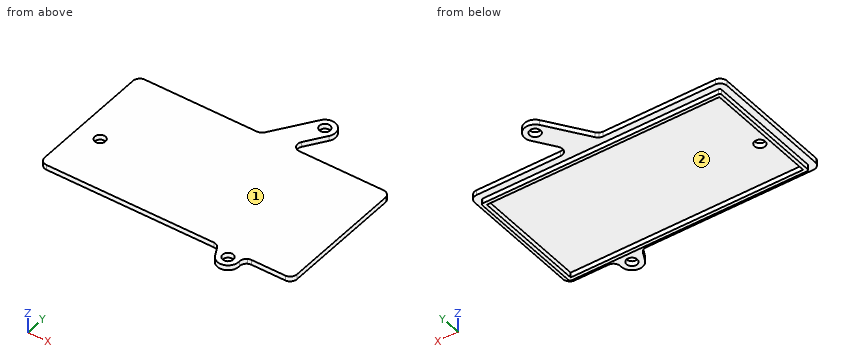
```python
from build123d import *

# Parameters (mm, degrees)
SKETCH1_W           = 69.1
SKETCH1_H           = 34.1
BOSS_EXTRUDE1_DEPTH = 1.5
BOSS_EXTRUDE2_DEPTH = 1.5
SKETCH3_R           = 1.6
BOSS_EXTRUDE3_DEPTH = 1.5
SKETCH3_2_R         = 1.6
CUT_EXTRUDE1_DEPTH  = 85.057646739


with BuildPart() as part:
    # Sketch1 → Boss-Extrude1 (new body)
    with BuildSketch(Plane.XY.offset(19)):
        with BuildLine():
            Line((4.325559412, 33.249665151), (-65.674440588, 33.249665151))
            ThreePointArc((-65.674440588, 33.249665151), (-66.063349318, 33.088573881), (-66.224440588, 32.699665151))
            Line((-66.224440588, 32.699665151), (-66.224440588, -2.300334849))
            ThreePointArc((-66.224440588, -2.300334849), (-66.063349318, -2.689243578), (-65.674440588, -2.850334849))
            Line((-65.674440588, -2.850334849), (4.325559412, -2.850334849))
            ThreePointArc((4.325559412, -2.850334849), (4.714468141, -2.689243578), (4.875559412, -2.300334849))
            Line((4.875559412, -2.300334849), (4.875559412, 32.699665151))
            ThreePointArc((4.875559412, 32.699665151), (4.714468141, 33.088573881), (4.325559412, 33.249665151))
        make_face()
        with Locations((-30.674440588, 15.199665151)):
            Rectangle(SKETCH1_W, SKETCH1_H, mode=Mode.SUBTRACT)
    extrude(amount=-BOSS_EXTRUDE1_DEPTH)

    # Sketch2 → Boss-Extrude2 (add)
    with BuildSketch(Plane.XY.offset(19)):
        with BuildLine():
            Line((6.825559412, -2.800334849), (6.825559412, 33.199665151))
            ThreePointArc((6.825559412, 33.199665151), (6.239772974, 34.613878714), (4.825559412, 35.199665151))
            Line((4.825559412, 35.199665151), (-66.174440588, 35.199665151))
            ThreePointArc((-66.174440588, 35.199665151), (-67.588654151, 34.613878714), (-68.174440588, 33.199665151))
            Line((-68.174440588, 33.199665151), (-68.174440588, -2.800334849))
            ThreePointArc((-68.174440588, -2.800334849), (-67.588654151, -4.214548411), (-66.174440588, -4.800334849))
            Line((-66.174440588, -4.800334849), (4.825559412, -4.800334849))
            ThreePointArc((4.825559412, -4.800334849), (6.239772974, -4.214548411), (6.825559412, -2.800334849))
        make_face()
    extrude(amount=BOSS_EXTRUDE2_DEPTH)

    # Sketch3 → Boss-Extrude3 (add)
    with BuildSketch(Plane.XY.offset(20.5)):
        with Locations((-61.556671003, 10.73089265)):
            Circle(SKETCH3_R)
        with BuildLine():
            Line((-14.637085978, -5.893524128), (-13.224518296, -8.670350201))
            ThreePointArc((-13.224518296, -8.670350201), (-9.526572542, -10.284819436), (-7.230629421, -6.966693625))
            ThreePointArc((-7.230629421, -6.966693625), (-7.001208277, -5.857177596), (-6.205806077, -5.050334849))
            ThreePointArc((-6.205806077, -5.050334849), (-5.737560241, -4.863843176), (-5.237560241, -4.800334849))
            Line((-5.237560241, -4.800334849), (-16.419694829, -4.800334849))
            ThreePointArc((-16.419694829, -4.800334849), (-15.919694829, -4.863843176), (-15.451448992, -5.050334849))
            ThreePointArc((-15.451448992, -5.050334849), (-14.981104401, -5.410925772), (-14.637085978, -5.893524128))
        make_face()
        with Locations((-10.394626745, -7.230788182)):
            Circle(SKETCH3_R, mode=Mode.SUBTRACT)
        with BuildLine():
            Line((-23.070638788, 47.711150724), (-31.122037847, 36.06249216))
            ThreePointArc((-31.122037847, 36.06249216), (-31.425094294, 35.716922893), (-31.799038979, 35.449665151))
            ThreePointArc((-31.799038979, 35.449665151), (-32.267284816, 35.263173478), (-32.767284816, 35.199665151))
            Line((-32.767284816, 35.199665151), (-20.185587119, 35.199665151))
            ThreePointArc((-20.185587119, 35.199665151), (-20.685587119, 35.263173478), (-21.153832956, 35.449665151))
            ThreePointArc((-21.153832956, 35.449665151), (-22.132771787, 36.743077954), (-21.830834088, 38.336838142))
            Line((-21.830834088, 38.336838142), (-17.846979662, 44.100626478))
            ThreePointArc((-17.846979662, 44.100626478), (-18.653547102, 48.517718164), (-23.070638788, 47.711150724))
        make_face()
        with Locations((-20.458809225, 45.905888601)):
            Circle(SKETCH3_R, mode=Mode.SUBTRACT)
    extrude(amount=-BOSS_EXTRUDE3_DEPTH)

    # Sketch3<2> → Cut-Extrude1 (cut, through all)
    with BuildSketch(Plane.XY.offset(20.5)):
        with Locations((-61.556671003, 10.73089265)):
            Circle(SKETCH3_2_R)
    extrude(amount=-CUT_EXTRUDE1_DEPTH, mode=Mode.SUBTRACT)


solid = part.part
```
Geometry: final body of the model. Coordinates: model frame, mm. Face numbers are marked on the shaded views. Give positions to 0.01 mm unless a question says otherwise; leave off trailing zeros. Order: outer loops, then holes, each group sorted by start corner. A loop starts at its lowest first (then second) coordinate and runs counter-clockwise, first axis right, second up. Notation, with made-up numbers: M 27,24.25 L 60,24.25 A13 cw 60,38.25 Z; hole C 52,78.25 d10. An arc over 180 degrees is marked long. Answer as CSV lines item,"result". Start each with the question number.
1) Cut plane C-C (x = -41). Output: boundary loops of the cut face in (y, z).
2) First-contact query: P1, Ø3.5, axis at x = -61.56, y = 10.73, coming from the -Z side; P2, Ø0.8, axis at x = -5.5, z = 20, coming from the +Y side; P3, Ø0.8, axis at x = -39.5, z = 19.5, coming from the -Y side. Flat tips, straight axial feed; report the tip coordinate or a pass-through.
3) Cut plane D-D (x = -11). Output: boundary loops of the cut face in (y, z).
4) Mould query, pull axis Y, two halves, no side actions, for the marked faces 1 and 2. Classes: +Y half, -Y half, draft (parallel to the pull), parting line (faces both ways), or undercut.
5) Cut plane A-A (z = 18.4). Output: boundary loops of the cut face in (x, y).
6) Line query: line 1 (Y direction, x = -38, z = 18.5); line 2 (X direction, y = 28, z = 18.3); line 3 (Z direction, x = -16, y = 21). Output: solid intervals per line, ascending. Write a range as from..to.
7) Cut plane B-B (y = 26). Output: boundary loops of the cut face in (x, z), then the cut area to 4 significant figures.
Findings below:
1,outline,"M -4.8,19 L -2.85,19 L -2.85,17.5 L -1.85,17.5 L -1.85,19 L 32.25,19 L 32.25,17.5 L 33.25,17.5 L 33.25,19 L 35.2,19 L 35.2,20.5 L -4.8,20.5 Z"
2,P1,"stops at z = 19"
2,P2,"stops at y = 35.2"
2,P3,"stops at y = -4.8"
3,outline,"M -10.35,19 L -8.71,19 L -8.71,20.5 L -10.35,20.5 Z; M -5.75,19 L -2.85,19 L -2.85,17.5 L -1.85,17.5 L -1.85,19 L 32.25,19 L 32.25,17.5 L 33.25,17.5 L 33.25,19 L 35.2,19 L 35.2,20.5 L -5.75,20.5 Z"
4,face 1,"draft"
4,face 2,"undercut"
5,outline,"M -66.22,-2.3 A0.55 ccw -65.67,-2.85 L 4.33,-2.85 A0.55 ccw 4.88,-2.3 L 4.88,32.7 A0.55 ccw 4.33,33.25 L -65.67,33.25 A0.55 ccw -66.22,32.7 Z; hole M -65.22,-1.85 L 3.88,-1.85 L 3.88,32.25 L -65.22,32.25 Z"
6,line 1,"y = -2.85..-1.85, 32.25..33.25"
6,line 2,"x = -66.22..-65.22, 3.88..4.88"
6,line 3,"z = 19..20.5"
7,outline,"M -68.17,19 L -66.22,19 L -66.22,17.5 L -65.22,17.5 L -65.22,19 L 3.88,19 L 3.88,17.5 L 4.88,17.5 L 4.88,19 L 6.83,19 L 6.83,20.5 L -68.17,20.5 Z"
7,area,"115.5 mm²"
